Could you check a few things on this drawing? It's one solid part, dimensions in mm from its lowest x, y, z. A direction names the side the tool comes from. Round coordinates to 2 decimals unless told otherwise and drop trailing zeros. Order: outer loops, then holes, each group sorted by start corner. A loop starts at its lowest first (then second) coordinate and runs counter-clockwise, first axis right, second up.
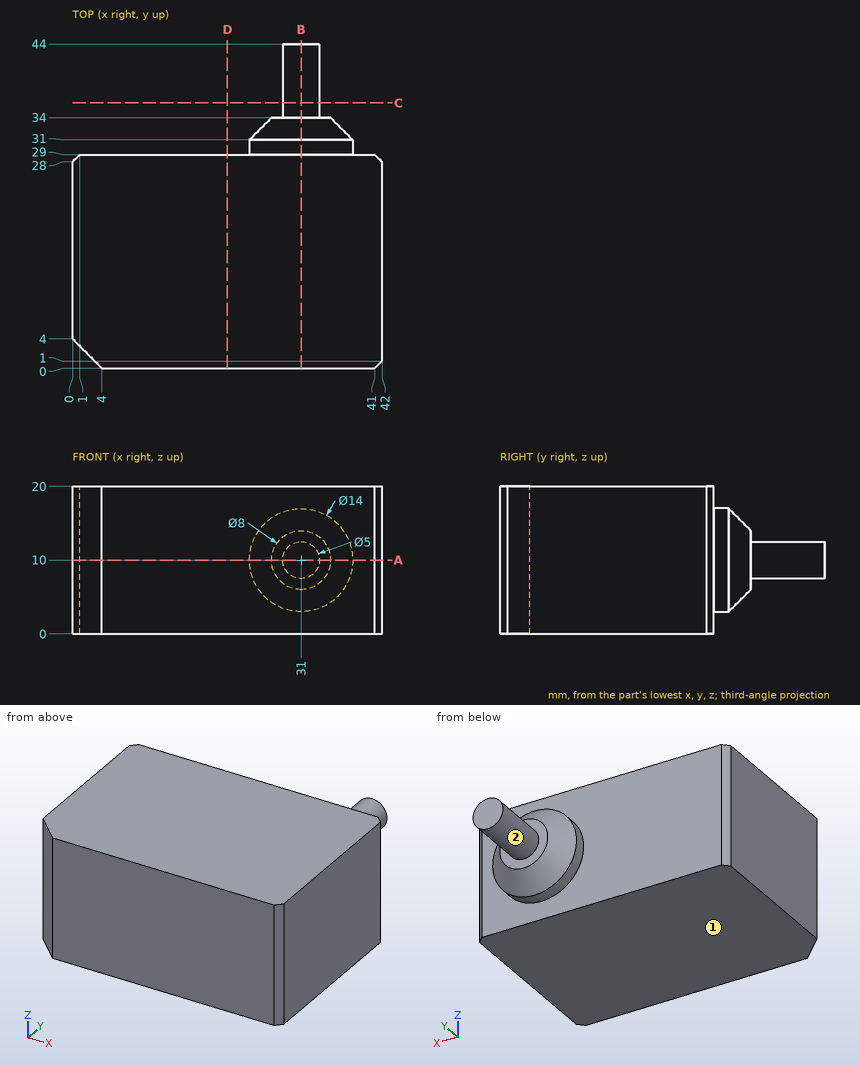
(1) I want a section at C-C, the plane y = 36. List the corners of the cut face in (x, z) for me, plus the area to 3 significant figures.
(2) I'm going to push a flat-ended pin straight in: pin 1 Ø4 at (x, z) = (13, 16) entering from +Y. Where does the tip first touch, or does it pass through?
(3) I want a section at D-D, the plane x = 21. List the corners of the cut face in (y, z) for me, plus the area to 3 significant figures.
(4) I want a section at A-A, the plane z = 10. List the corners of the cut face in (x, y) for me.
(5) Please list where these lines run through material, in increasing order: probe 1 along Y at (x, z) = (8.5, 17); probe 2 along Y at (x, z) = (35, 4.5); probe 3 along X at (y, z) = (42, 8).
(6) I want a section at B-B, the plane x = 31. List the corners of the cut face in (y, z) for me, plus the area to 3 significant figures.
(7) On a 3-axis mill with a long thin cutter (end or side, diameter ignored), from which of +Z, -Z, +X, -X, +Y, -Y can I reach the whole of each face in a straight line? I mean the marked faces 1 and 2. Say none if no direction works.
Ans:
1. outline: circle Ø5 at (31, 10)
1. area: 19.6 mm2
2. pin 1: stops at y = 29
3. outline: (0, 0) - (29, 0) - (29, 20) - (0, 20) - close
3. area: 580 mm2
4. outline: (0, 4) - (4, 0) - (41, 0) - (42, 1) - (42, 28) - (41, 29) - (38, 29) - (38, 31) - (35, 34) - (33.5, 34) - (33.5, 44) - (28.5, 44) - (28.5, 34) - (27, 34) - (24, 31) - (24, 29) - (1, 29) - (0, 28) - close
5. probe 1: y = 0 to 29
5. probe 2: y = 0 to 31.2
5. probe 3: x = 29.5 to 32.5
6. outline: (0, 0) - (29, 0) - (29, 3) - (31, 3) - (34, 6) - (34, 7.5) - (44, 7.5) - (44, 12.5) - (34, 12.5) - (34, 14) - (31, 17) - (29, 17) - (29, 20) - (0, 20) - close
6. area: 691 mm2
7. face 1: -Z, +X, -X, +Y, -Y
7. face 2: +Y
